from build123d import *

# Parameters (mm, degrees)
F0_R     = 50
F1_DEPTH = 15
F2_R     = 7
F3_R     = 7
F5_DEPTH = 42.6


with BuildPart() as f1:
    # F0 (on Front) → F1 (new body)
    with BuildSketch(Plane.XZ):
        with BuildLine():
            Line((-13.692577, 94.988603), (-13.692577, 73.739497))
            ThreePointArc((-13.692577, 73.739497), (-51.872276, 54.168874), (-73.077535, 16.872283))
            Line((-73.077535, 16.872283), (-93.077535, 16.872283))
            Line((-93.077535, 16.872283), (-93.077535, 6.872283))
            Line((-93.077535, 6.872283), (-68.077535, 6.872283))
            Line((-68.077535, 6.872283), (-68.077535, -13.127717))
            Line((-68.077535, -13.127717), (-93.077535, -13.127717))
            Line((-93.077535, -13.127717), (-93.077535, -23.127717))
            Line((-93.077535, -23.127717), (-71.344998, -23.127717))
            ThreePointArc((-71.344998, -23.127717), (-47.086109, -58.377207), (-7.5, -74.624058))
            Line((-7.5, -74.624058), (-7.5, -94.624058))
            Line((-7.5, -94.624058), (0, -94.624058))
            Line((0, -94.624058), (7.5, -94.624058))
            Line((7.5, -94.624058), (7.5, -74.624058))
            ThreePointArc((7.5, -74.624058), (74.935838, 3.101649), (1.307423, 74.988603))
            Line((1.307423, 74.988603), (1.307423, 94.988603))
            Line((1.307423, 94.988603), (-6.192577, 94.988603))
            Line((-6.192577, 94.988603), (-13.692577, 94.988603))
        make_face()
        Circle(F0_R, mode=Mode.SUBTRACT)
    extrude(amount=F1_DEPTH)

    # F2
    f2_edges = [f1.edges().sort_by_distance(p)[0] for p in [
        (-7.5, -15, -84.624058),
        (7.5, -15, -84.624058),
        (7.5, 0, -84.624058),
        (-7.5, 0, -84.624058),
    ]]
    fillet(f2_edges, radius=F2_R)

    # F3
    f3_edges = [f1.edges().sort_by_distance(p)[0] for p in [
        (1.307423, -15, 84.988603),
        (1.307423, 0, 84.988603),
        (-13.692577, -15, 84.36405),
        (-13.692577, 0, 84.36405),
    ]]
    fillet(f3_edges, radius=F3_R)

    # F4 (on face) → F5 (cut)
    with BuildSketch(Plane.XY.offset(16.872283)):
        with BuildLine():
            ThreePointArc((-89.077535, -7.5), (-83.077535, -13.5), (-77.077535, -7.5))
            ThreePointArc((-77.077535, -7.5), (-83.077535, -1.5), (-89.077535, -7.5))
        make_face()
    extrude(amount=-F5_DEPTH, mode=Mode.SUBTRACT)


solid = f1.part
Verification items for the finished model (mm, model axes). A direction names the side the tool comes from. Give positions to 0.01 mm unless a question says otherwise; leave off trailing zeros. Write each loop counter-clockwise with the first axis right and the second up, starting at its lowest first coordinate (ties: lowest second). Pieces come first, ordered by that corner, then holes. Notation, with made-up numbers: (58, -39.5) -> (98, -39.5) arc R9 cw to (98, -22.5) -> close; hole circle Ø6 at (58, 45). An arc over 180 degrees is marked (long way). Use CSV: the item, a comma, the result in double quotes.
(1) Sectioned sample at C-C (y = -4.5). Record the cut outline in (x, z) (3 decimals).
Derived:
outline,"(-93.078, -23.128) -> (-88.274, -23.128) -> (-88.274, -13.128) -> (-93.078, -13.128) -> close; (-93.078, 6.872) -> (-88.274, 6.872) -> (-88.274, 16.872) -> (-93.078, 16.872) -> close; (-77.881, -23.128) -> (-71.345, -23.128) arc R75 ccw to (-7.038, -74.669) -> (-7.038, -94.624) -> (7.038, -94.624) -> (7.038, -74.669) arc R75 ccw to (0.846, 74.995) -> (0.846, 94.989) -> (-13.231, 94.989) -> (-13.231, 73.824) arc R75 ccw to (-73.078, 16.872) -> (-77.881, 16.872) -> (-77.881, 6.872) -> (-68.078, 6.872) -> (-68.078, -13.128) -> (-77.881, -13.128) -> close; hole circle Ø100 at (0, 0)"
(2) Sectioned sample at A-A (z = 0). Record the cut outline in (x, y).
Derived:
outline,"(-68.08, -15) -> (-50, -15) -> (-50, 0) -> (-68.08, 0) -> close; (50, -15) -> (75, -15) -> (75, 0) -> (50, 0) -> close"
(3) Material ranges on L1, parallel to X at y = -11.25, z = -20.5; L2, parallel to Z at x = 0, y = -3.5; L3, parallel to X at y = -9.75, z = 36, recorded low to high.
Derived:
L1,"x = -93.08 to -87.76, -78.39 to -45.6, 45.6 to 72.14"
L2,"z = -94.62 to -50, 50 to 94.99"
L3,"x = -65.8 to -34.7, 34.7 to 65.8"
(4) Sectioned sample at B-B (x = -41.5). Record the cut outline in (y, z), plus the area to 3 significant figures.
Derived:
outline,"(-15, -62.47) -> (0, -62.47) -> (0, -27.89) -> (-15, -27.89) -> close; (-15, 27.89) -> (0, 27.89) -> (0, 62.47) -> (-15, 62.47) -> close"
area,"1,040 mm^2"
(5) Release check for a two-part mould opening along X. For faces 1 (the cylindrical face through (-5.5, -2.1, -84.8)), 2 (the cylindrical face through (-89.07, -7.24, -18.06)), 3 (the cylindrical face through (5.5, -2.1, -84.5)) record: +X half, -X half, draft (parallel to the pull), parting line (faces both ways), or undercut.
Derived:
face 1,"-X half"
face 2,"undercut"
face 3,"+X half"
(6) Sectioned sample at D-D (x = 53). Record the cut outline in (y, z), plus the area to 3 significant figures.
Derived:
outline,"(-15, -53.07) -> (0, -53.07) -> (0, 53.07) -> (-15, 53.07) -> close"
area,"1,590 mm^2"
(7) Set-up check for faces 4 (the cylindrical face through (-5.5, -12.9, -84.8)), 5 (the cylindrical face through (-0.798, -1.996, 85.028)), 6 (the cylindrical face through (-11.696, -12.895, 84.215)): record each of +Z, -Z, +X, -X, +Y, -Y from which the full face is reachable in a straight line by a thin tool's end or side.
Derived:
face 4,"-Z, -X, -Y"
face 5,"+Z, +X, +Y"
face 6,"+Z, -X, -Y"
(8) Go/stop test with flat-tipped pins: pin 1 (1 mm diameter, centred on x = -33, y = -2, fed in from +Z); pin 2 (0.8 mm diameter, centred on y = -7.5, z = 87.5, fed in from +X); pin 3 (2 mm diameter, centred on x = 53.5, y = -7, fed in from +Z). Record where each tip stops, or that it passes through.
Derived:
pin 1,"stops at z = 67.59"
pin 2,"stops at x = 1.31"
pin 3,"stops at z = 53.56"
